from build123d import *

# Parameters (mm, degrees)
SKETCH11_R                   = 3.1
EXTRUDE1_DEPTH               = 12
M6_TAPPED_HOLE1_D            = 5
M6_TAPPED_HOLE1_DEPTH        = 35
M6_TAPPED_HOLE1_TIP          = 1.502151548
F_7_0_7_DIAMETER_HOLE1_D     = 7
F_7_0_7_DIAMETER_HOLE1_DEPTH = 4
F_7_0_7_DIAMETER_HOLE1_TIP   = 2.103012167
EXTRUDE3_DEPTH               = 1


with BuildPart() as part:
    # Sketch1 → Revolve1 (revolve)
    with BuildSketch(Plane.XY, mode=Mode.PRIVATE) as revolve1_sk:
        Polygon((8, 18.5), (0, 15), (0, 8.5675), (20.675, 6.5), (22, 7.825), (32, 7.825), (32, 21.5), (8, 21.5), align=None)
    revolve(revolve1_sk.sketch.rotate(Axis((0, 0, 0), (1, 0, 0)), 90), axis=Axis((0, 0, 0), (1, 0, 0)))

    # Sketch11 → Extrude1 (cut)
    with BuildSketch(Plane(origin=(32, 0, 0), x_dir=(0, 0, -1), z_dir=(1, 0, 0))):
        with Locations((0, -17)):
            Circle(SKETCH11_R)
        with Locations((-14.722431864, -8.5)):
            Circle(SKETCH11_R)
        with Locations((-14.722431864, 8.5)):
            Circle(SKETCH11_R)
        with Locations((0, 17)):
            Circle(SKETCH11_R)
        with Locations((14.722431864, 8.5)):
            Circle(SKETCH11_R)
        with Locations((14.722431864, -8.5)):
            Circle(SKETCH11_R)
    extrude(amount=-EXTRUDE1_DEPTH, mode=Mode.SUBTRACT)

    # M6 Tapped Hole1
    with Locations(Plane(origin=(20, -17, 0), x_dir=(0, 0, 1), z_dir=(1, 0, 0))):
        with Locations((0, 0), (14.722431864, -8.5), (14.722431864, -25.5), (0, -34), (-14.722431864, -25.5), (-14.722431864, -8.5)):
            Hole(M6_TAPPED_HOLE1_D / 2, depth=M6_TAPPED_HOLE1_DEPTH)
            with Locations((0, 0, -(M6_TAPPED_HOLE1_DEPTH + M6_TAPPED_HOLE1_TIP / 2))):  # 118° drill point
                Cone(0, M6_TAPPED_HOLE1_D / 2, M6_TAPPED_HOLE1_TIP, mode=Mode.SUBTRACT)

    # Ø7.0 (7) Diameter Hole1
    with Locations(Plane(origin=(32, -13.856406461, -8), x_dir=(0, 0, 1), z_dir=(1, 0, 0))):
        with Locations((0, 0), (16, 0), (24, -13.856406461), (16, -27.712812922), (0, -27.712812922), (-8, -13.856406461)):
            Hole(F_7_0_7_DIAMETER_HOLE1_D / 2, depth=F_7_0_7_DIAMETER_HOLE1_DEPTH)
            with Locations((0, 0, -(F_7_0_7_DIAMETER_HOLE1_DEPTH + F_7_0_7_DIAMETER_HOLE1_TIP / 2))):  # 118° drill point
                Cone(0, F_7_0_7_DIAMETER_HOLE1_D / 2, F_7_0_7_DIAMETER_HOLE1_TIP, mode=Mode.SUBTRACT)

    # Sketch18 → Extrude3 (cut, symmetric)
    with BuildSketch(Plane.XY):
        Polygon((23.570558224, 5.305955372), (-1.084590537, 7.771470248), (-0.78607938, 10.756581818), (23.869069381, 8.291066942), align=None)
    extrude(amount=EXTRUDE3_DEPTH, both=True, mode=Mode.SUBTRACT)


solid = part.part
Build history of the part. All positions in model axes, mm. A direction names the side the tool comes from. Give positions to 0.01 mm unless a question says otherwise; leave off trailing zeros. Loops run counter-clockwise (first coordinate to the right, second up) from the corner with the lowest first, then second, coordinate; pieces in that order, holes last. Notation, with made-up numbers: (74, 58.25) - (124, 58.25) arc R10 cw to (124, 67.25) - close; hole circle Ø5 at (51.5, 49). An arc over 180 degrees is marked (long way). Write item = value, one per line. Start each with the question number.
1) Band-saw the part on B-B on y = 9.5. Count the separate pieces of the cut face and the enclosed holes in it, plus the area to 3 significant figures.
2) Drop flat-ended pins along their axis: pin 1 Ø4.5 at (y, z) = (-8.5, -14.72) entering from +X; pin 2 Ø6 at (x, z) = (9, 15.5) entering from -Y; pin 3 Ø2 at (x, z) = (24.5, -16.5) entering from +Y; pin 4 Ø2 at (x, z) = (13, 7.5) entering from -Y. Give the stop position or say it passes through.
3) Tool access for faces 4 (the cylindrical face through (29.972, 15.986, -5.223)), 5 (the conical face through (3.944, 0.101, 16.725)): list every direction of +Z, -Z, +X, -X, +Y, -Y with a clear straight run to the whole face (end or side of a thin tool).
4) Pull direction Y, two halves, no side cores. Call faces 1 (the flat face through (20, -8, -12)), 2 (the flat face through (0, 6.4, 6.5)), 3 (the conical face through (3.9, 14.5, 8.3)): +Y half, -Y half, draft (parallel to the pull), parting line (faces both ways), or undercut.
5) Band-saw the part on A-A on x = 12. Give the cut face in (y, z) (1 decimal).
6) Probe probe 1 along Z at (x, y) = (21.5, -6.5); probe 2 along Y at (x, z) = (24, -15); probe 3 along Y at (x, z) = (29.7, -8). List the from-to ranges inside material, lowest first. Write a range as from..to.
Final values:
q1.separate_pieces = 3
q1.enclosed_holes = 0
q1.area = 849 mm²
q2.pin_1 = through
q2.pin_2 = -17.49
q2.pin_3 = 14.9
q2.pin_4 = -20.49
q3.face_4 = +X
q3.face_5 = +Z, -X
q4.face_1 = undercut
q4.face_2 = draft
q4.face_3 = +Y half
q5.outline = circle Ø43 at (0, 0); hole circle Ø5 at (-17, 0); hole circle Ø5 at (-8.5, -14.7); hole circle Ø5 at (-8.5, 14.7); hole circle Ø5 at (8.5, -14.7); hole circle Ø5 at (8.5, 14.7); hole (7.3, -1) - (9.5, -1) - (9.5, 1) - (7.3, 1) arc R7.4 ccw (long way) to start; hole circle Ø5 at (17, 0)
q6.probe_1 = -20.49..-17.09, -12.35..-3.38, 3.38..12.35, 17.09..20.49
q6.probe_2 = -15.4..-11.59, -5.41..5.41, 11.59..15.4
q6.probe_3 = -19.96..-17.36, -10.36..10.36, 17.36..19.96
